Geometry check sheet. Reference: the model listing, model coordinates, mm. Face numbers are marked on the shaded views. Give positions to 0.01 mm unless a question says otherwise; leave off trailing zeros. Order: outer loops, then holes, each group sorted by start corner. A loop starts at its lowest first (then second) coordinate and runs counter-clockwise, first axis right, second up. Notation, with made-up numbers: M -24.75,-22 L -16.75,-22 A10 cw -16.75,-16 Z; hole C -1.5,-29.75 d3. An arc over 180 degrees is marked long. Put each result on its own line as item: value. Start each with the question number.
Q1. Mould release check, pull along Z, two halves, no side actions. Record for the marked faces 1, 2, 3 and 4: +Z half, -Z half, draft (parallel to the pull), parting line (faces both ways), or undercut.
Q2. Section check C-C on y = 12.25. Record the cut outline in (x, z) (1 decimal), then the cut area to 3 significant figures.
Q3. Material ranges on L1, parallel to Z at x = -72.5, y = 19.5; L2, parallel to Z at x = -10, y = 3.75 (3 decimals); L3, parallel to X at y = 6.5, z = 3, recorded low to high.
Q4. Section check B-B on z = 16. Record the cut outline in (x, y).
Q5. Section check A-A on x = -6.5. Record the cut outline in (y, z) (3 decimals), then the cut area to 3 significant figures.
Q6. Section check D-D on z = 23. Record the cut outline in (x, y).
Autodesk Inventor part; units mm, degrees
ref_plane "YZ Plane" through (0, 0, 0) normal (1, 0, 0) x (0, 1, 0)
ref_plane "XZ Plane" through (0, 0, 0) normal (0, 1, 0) x (-1, 0, 0)
ref_plane "XY Plane" through (0, 0, 0) normal (0, 0, 1) x (1, 0, 0)
sketch "Sketch1" plane through (0, 0, 0) normal (0, 1, 0) x (-1, 0, 0)
  line L0 (0, 0) -> (112, 0)
  line L1 (112, 0) -> (112, 40.005)
  line L2 (112, 40.005) -> (0, 40.005)
  line L3 (0, 40.005) -> (0, 0)
  dimension "d0" = 112
  dimension "d1" = 40.005
extrude "Extrusion1" add sketch "Sketch1" along normal blind 20.32
sketch "Sketch2" plane through (0, 20.32, 0) normal (0, 1, 0) x (1, 0, 0)
  line L0 (-112, 0) -> (-112, -40.005)
  line L1 (0, -40.005) -> (0, 0)
  line L2 (-112, -20.0025) -> (-102.5004, -20.0025) construction
  line L3 (0, -20.0025) -> (-9.4996, -20.0025) construction
  circle A0 centre (-9.4996, -20.0025) radius 5
  circle A1 centre (-102.5004, -20.0025) radius 5
  dimension "d4" = 9.4996
  dimension "d5" = 9.4996
  dimension "d6" = 10
  dimension "d7" = 10
extrude "Extrusion2" cut sketch "Sketch2" against normal blind 20.32
fillet "Fillet1" radius 4 4 edges at (-112, 10.16, 40.005) (-112, 10.16, 0) (0, 10.16, 40.005) (0, 10.16, 0)
fillet "Fillet2" radius 1 16 edges at (-110.8284, 0, 1.1716) (-112, 0, 20.0025) (-110.8284, 0, 38.8334) (-56, 0, 40.005) (-1.1716, 0, 38.8334) (0, 0, 20.0025) (-1.1716, 0, 1.1716) (-56, 0, 0) (-110.8284, 20.32, 1.1716) (-112, 20.32, 20.0025) (-110.8284, 20.32, 38.8334) (-56, 20.32, 40.005) (-1.1716, 20.32, 38.8334) (0, 20.32, 20.0025) (-1.1716, 20.32, 1.1716) (-56, 20.32, 0)
equation "\"d5\" = d4"
properties part number "CIM Mount Top" material "Aluminum 6061"
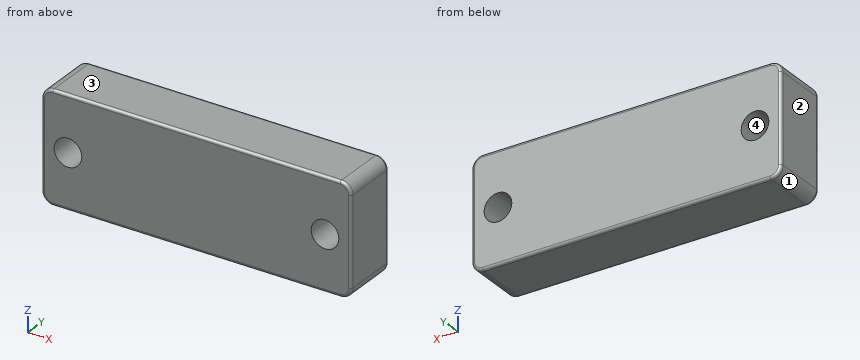
Results found:
1. face 1: -Z half
1. face 2: draft
1. face 3: +Z half
1. face 4: undercut
2. outline: M -112,4 A4 ccw -108,0 L -4,0 A4 ccw 0,4 L 0,36 A4 ccw -4,40 L -108,40 A4 ccw -112,36 Z; hole C -102.5,20 d10; hole C -9.5,20 d10
2. area: 4,310 mm^2
3. L1: z = 0.02 to 39.99
3. L2: z = 0 to 15.028, 24.977 to 40.005
3. L3: x = -111.87 to -0.13
4. outline: M -112,1 A1 ccw -111,0 L -105.5,0 L -105.5,20.32 L -111,20.32 A1 ccw -112,19.32 Z; M -99.5,0 L -12.5,0 L -12.5,20.32 L -99.5,20.32 Z; M -6.5,0 L -1,0 A1 ccw 0,1 L 0,19.32 A1 ccw -1,20.32 L -6.5,20.32 Z
5. outline: M 0,1 A1 ccw 1,0 L 19.32,0 A1 ccw 20.32,1 L 20.32,16.002 L 0,16.002 Z; M 0,24.003 L 20.32,24.003 L 20.32,39.005 A1 ccw 19.32,40.005 L 1,40.005 A1 ccw 0,39.005 Z
5. area: 649 mm^2
6. outline: M -112,1 A1 ccw -111,0 L -106.5,0 L -106.5,20.32 L -111,20.32 A1 ccw -112,19.32 Z; M -98.5,0 L -13.5,0 L -13.5,20.32 L -98.5,20.32 Z; M -5.5,0 L -1,0 A1 ccw 0,1 L 0,19.32 A1 ccw -1,20.32 L -5.5,20.32 Z
